CAD build for the part. Positions are in the model's coordinates, mm. Face numbers are marked on the shaded views. Coordinates: 2 decimals unless noted, no trailing zeros. Loops run counter-clockwise (first coordinate to the right, second up) from the corner with the lowest first, then second, coordinate; pieces in that order, holes last. Notation, with made-up numbers: (18, -9.75) -> (51, -9.75) arc R12 cw to (51, 7.25) -> close; hole circle Ø5 at (-4, -38.75). An arc over 180 degrees is marked (long way). Answer as a JSON object with one key per item and string values. Group by question number.
from build123d import *

# Parameters (mm, degrees)
CYLINDER001_R     = 8.5
CYLINDER001_DEPTH = 10
CYLINDER_R        = 10
CYLINDER_DEPTH    = 2
CYLINDER002_R     = 2
CYLINDER002_DEPTH = 2


with BuildPart() as cilindro001:
    # Cylinder001 → Cylinder001 (new body)
    with BuildSketch(Plane.XY.offset(-4)):
        Circle(CYLINDER001_R)
    extrude(amount=CYLINDER001_DEPTH)


with BuildPart() as cut:
    # Cylinder → Cylinder (new body)
    with BuildSketch(Plane.XY):
        Circle(CYLINDER_R)
    extrude(amount=CYLINDER_DEPTH)

    # Cut: cut Cilindro001
    add(cilindro001.part, mode=Mode.SUBTRACT)


with BuildPart() as obj1:
    # Cylinder002 → Cylinder002 (new body)
    with BuildSketch(Plane(origin=(-7.4, 8.4, 0), x_dir=(1, 0, 0), z_dir=(0, 0, 1))):
        Circle(CYLINDER002_R)
    extrude(amount=CYLINDER002_DEPTH)


with BuildPart() as part_mirroring:
    # Part__Mirroring: instance of obj1
    add(obj1.part.mirror(Plane(origin=(0, 0, 0), x_dir=(0, -1, 0), z_dir=(1, 0, 0))))


with BuildPart() as obj2:
    # Fusion base: copy of obj1
    add(obj1.part)

    # Fusion: union Part__Mirroring
    add(part_mirroring.part)

    # Fusion001: union Cut
    add(cut.part)


solid = obj2.part
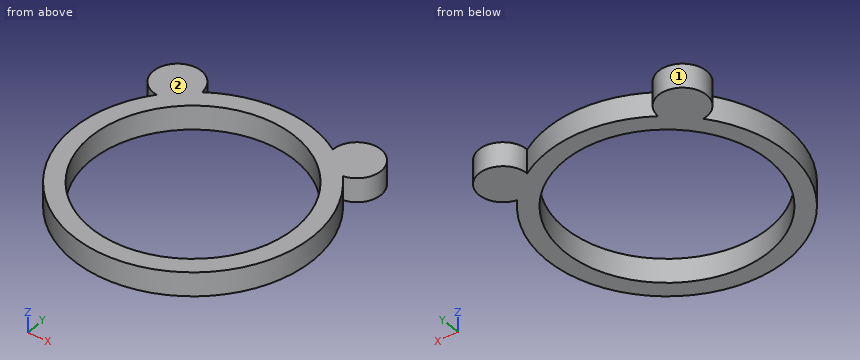
Item 1: Drill centre lines: L1, parallel to X at y = 0, z = 1.6; L2, parallel to X at y = 6.75, z = 1.8. Where is each one in solid material? Low to high.
Item 2: Pull direction Y, two halves, no side cores. Call the marked faces 1 and 2: +Y half, -Y half, draft (parallel to the pull), parting line (faces both ways), or undercut.
Item 3: Band-saw the part on C-C, the plane x = -6.25. List the corners of the cut face in (y, z), and give its area (3 significant figures).
Item 4: Band-saw the part on B-B, the plane y = 0. List the corners of the cut face in (x, z).
Item 5: Band-saw the part on A-A, the plane x = 8. List the corners of the cut face in (y, z), and give its area (3 significant figures).
Item 6: Band-saw the part on D-D, the plane y = 9. List the corners of the cut face in (x, z).
Reply:
{
 "1": {"L1": "-10 to -8.5, 8.5 to 10", "L2": "-8.53 to -5.17, 5.17 to 8.53"},
 "2": {"face 1": "undercut", "face 2": "draft"},
 "3": {"outline": "(-7.81, 0) -> (-5.76, 0) -> (-5.76, 2) -> (-7.81, 2) -> close; (5.76, 0) -> (10.04, 0) -> (10.04, 2) -> (5.76, 2) -> close", "area": "12.6 mm²"},
 "4": {"outline": "(-10, 0) -> (-8.5, 0) -> (-8.5, 2) -> (-10, 2) -> close; (8.5, 0) -> (10, 0) -> (10, 2) -> (8.5, 2) -> close"},
 "5": {"outline": "(-6, 0) -> (-2.87, 0) -> (-2.87, 2) -> (-6, 2) -> close; (2.87, 0) -> (6, 0) -> (6, 2) -> (2.87, 2) -> close; (6.49, 0) -> (10.31, 0) -> (10.31, 2) -> (6.49, 2) -> close", "area": "20.1 mm²"},
 "6": {"outline": "(-9.31, 0) -> (-5.49, 0) -> (-5.49, 2) -> (-9.31, 2) -> close; (-4.36, 0) -> (4.36, 0) -> (4.36, 2) -> (-4.36, 2) -> close; (5.49, 0) -> (9.31, 0) -> (9.31, 2) -> (5.49, 2) -> close"}
}
